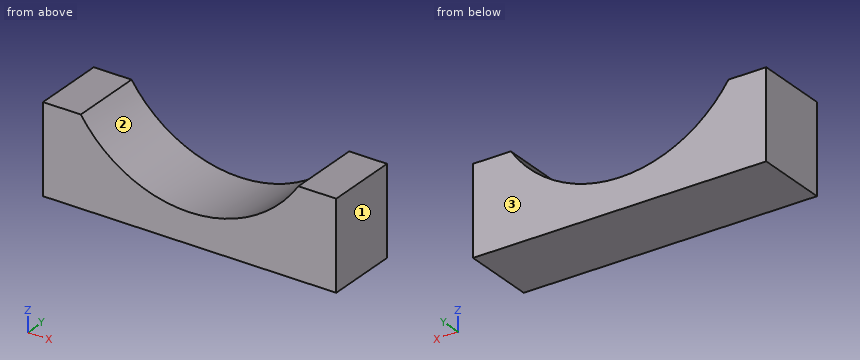
```python
from build123d import *

# Parameters (mm, degrees)
F1_DEPTH = 50


with BuildPart() as f1:
    # F0 (on Front) → F1 (new body)
    with BuildSketch(Plane.XZ):
        with BuildLine():
            ThreePointArc((74.231058, -50), (0, -89.5), (-74.231058, -50))
            Line((-74.231058, -50), (-100, -50))
            Line((-100, -50), (-100, -110))
            Line((-100, -110), (100, -110))
            Line((100, -110), (100, -50))
            Line((100, -50), (74.231058, -50))
        make_face()
    extrude(amount=-F1_DEPTH)


solid = f1.part
```
CAD build for the part. Positions are in the model's coordinates, mm. Face numbers are marked on the shaded views. Round coordinates to 2 decimals unless told otherwise and drop trailing zeros. Write each loop counter-clockwise with the first axis right and the second up, starting at its lowest first coordinate (ties: lowest second). Pieces come first, ordered by that corner, then holes.
Item 1: Mould opens along X. For the marked faces 1, 2 and 3 say: released by +X, released by -X, zero draft, split by the parting line, or undercut.
Filled in:
face 1: released by +X
face 2: undercut
face 3: zero draft
Item 2: Band-saw the part on A-A on z = -65.5. Write the cut outline in (x, y), then the cut area to 3 significant figures.
Filled in:
outline: (-100, 0) - (-60.99, 0) - (-60.99, 50) - (-100, 50) - close; (60.99, 0) - (100, 0) - (100, 50) - (60.99, 50) - close
area: 3,900 mm2
Item 3: Band-saw the part on D-D on x = 18. Write the cut outline in (y, z), then the cut area to 3 significant figures.
Filled in:
outline: (0, -110) - (50, -110) - (50, -87.67) - (0, -87.67) - close
area: 1,120 mm2
Item 4: Band-saw the part on B-B on y = 19.5. Write the cut outline in (x, z).
Filled in:
outline: (-100, -110) - (100, -110) - (100, -50) - (74.23, -50) arc R89.5 cw to (-74.23, -50) - (-100, -50) - close
Item 5: Drop a flat-ended pin along its axis: pin 1 Ø1 at (x, y) = (-44, 15.5) entering from +Z. Give the stop position or say it passes through.
Filled in:
pin 1: stops at z = -77.65
Item 6: Band-saw the part on C-C on z = -74. Write the cut outline in (x, y).
Filled in:
outline: (-100, 0) - (-50.34, 0) - (-50.34, 50) - (-100, 50) - close; (50.34, 0) - (100, 0) - (100, 50) - (50.34, 50) - close
Item 7: Drill centre lines: L1, parallel to X at y = 23, z = -60; L2, parallel to X at y = 19, z = -70; L3, parallel to Z at x = -49, y = 42. Where is each one in solid material? Low to high.
Filled in:
L1: x = -100 to -66.41, 66.41 to 100
L2: x = -100 to -55.77, 55.77 to 100
L3: z = -110 to -74.89
